Geometry check sheet. Reference: the model listing, model coordinates, mm. Give positions to 0.01 mm unless a question says otherwise; leave off trailing zeros. Loops run counter-clockwise (first coordinate to the right, second up) from the corner with the lowest first, then second, coordinate; pieces in that order, holes last.
1. Cross-section at C-C, the plane x = 16.5. Record the cut outline in (y, z), plus the area to 3 significant figures.
2. Cross-section at A-A, the plane y = 11. Record the cut outline in (x, z), plus the area to 3 significant figures.
3. Cross-section at B-B, the plane x = 28. Record the cut outline in (y, z).
4. Release check for a two-part mould opening along Y. For faces 1 (the cylindrical face through (28.378, 21.699, 4.715)), 2 (the flat face through (27.6, 13.4, 5)), 3 (the flat face through (28, 0, 2)), 4 (the cylindrical face through (39.24, 12.983, 2.535)) record: +Y half, -Y half, draft (parallel to the pull), parting line (faces both ways), or undercut.
5. Material ranges on L1, parallel to Y at x = 16.5, z = 1.45; L2, parallel to X at y = 10.5, z = 3.3; L3, parallel to Y at x = 6, z = 4.1, recorded low to high.
6. Cross-section at D-D, the plane x = 40.5. Record the cut outline in (y, z).
from build123d import *

# Parameters (mm, degrees)
SKETCH_BASE_W                                   = 56
SKETCH_BASE_H                                   = 22
BASE_EXTRUDE_DEPTH                              = 5
SKETCH2_R                                       = 2
MOUNTING_HOLES_DEPTH                            = 61.373835392
SMALL_EDGE_FILLET_R                             = 1
FILLET4_R                                       = 1
CSK_FOR_M4_FLAT_HEAD_MACHINE_SCREW4_D           = 4.3
CSK_FOR_M4_FLAT_HEAD_MACHINE_SCREW4_CSINK_D     = 9.4
CSK_FOR_M4_FLAT_HEAD_MACHINE_SCREW4_CSINK_ANGLE = 90


with BuildPart() as part:
    # Sketch-Base → Base-Extrude (new body)
    with BuildSketch(Plane.XY):
        with Locations((28, 11)):
            Rectangle(SKETCH_BASE_W, SKETCH_BASE_H)
    extrude(amount=BASE_EXTRUDE_DEPTH)

    # Sketch2 → Mounting Holes (cut, through all)
    with BuildSketch(Plane.XY.offset(5)):
        with Locations((16.5, 11)):
            Circle(SKETCH2_R)
        with Locations((39.5, 11)):
            Circle(SKETCH2_R)
    extrude(amount=-MOUNTING_HOLES_DEPTH, mode=Mode.SUBTRACT)

    # Small Edge Fillet
    small_edge_fillet_edges = [part.edges().sort_by_distance(p)[0] for p in [
        (0, 22, 2.5),
        (56, 22, 2.5),
        (56, 0, 2.5),
        (0, 0, 2.5),
    ]]
    fillet(small_edge_fillet_edges, radius=SMALL_EDGE_FILLET_R)

    # Fillet4
    fillet4_edges = [part.edges().sort_by_distance(p)[0] for p in [
        (28, 22, 0),
        (28, 22, 5),
        (0, 11, 0),
        (56, 11, 0),
        (28, 0, 0),
        (0.292893219, 21.707106781, 0),
        (0.292893219, 0.292893219, 0),
        (55.707106781, 0.292893219, 0),
        (55.707106781, 21.707106781, 0),
        (56, 11, 5),
        (0, 11, 5),
        (28, 0, 5),
        (0.292893219, 21.707106781, 5),
        (0.292893219, 0.292893219, 5),
        (55.707106781, 0.292893219, 5),
        (55.707106781, 21.707106781, 5),
    ]]
    fillet(fillet4_edges, radius=FILLET4_R)

    # CSK for M4 Flat Head Machine Screw4 (through all)
    with Locations(Plane(origin=(28, 11, 0), x_dir=(-1, 0, 0), z_dir=(0, 0, -1))):
        with Locations((0, 0)):
            CounterSinkHole(CSK_FOR_M4_FLAT_HEAD_MACHINE_SCREW4_D / 2, CSK_FOR_M4_FLAT_HEAD_MACHINE_SCREW4_CSINK_D / 2, counter_sink_angle=CSK_FOR_M4_FLAT_HEAD_MACHINE_SCREW4_CSINK_ANGLE)


solid = part.part
Result:
1. outline: (0, 1) arc R1 ccw to (1, 0) - (9, 0) - (9, 5) - (1, 5) arc R1 ccw to (0, 4) - close; (13, 0) - (21, 0) arc R1 ccw to (22, 1) - (22, 4) arc R1 ccw to (21, 5) - (13, 5) - close
1. area: 89.1 mm2
2. outline: (0, 1) arc R1 ccw to (1, 0) - (14.5, 0) - (14.5, 5) - (1, 5) arc R1 ccw to (0, 4) - close; (18.5, 0) - (23.3, 0) - (25.85, 2.55) - (25.85, 5) - (18.5, 5) - close; (30.15, 2.55) - (32.7, 0) - (37.5, 0) - (37.5, 5) - (30.15, 5) - close; (41.5, 0) - (55, 0) arc R1 ccw to (56, 1) - (56, 4) arc R1 ccw to (55, 5) - (41.5, 5) - close
2. area: 211 mm2
3. outline: (0, 1) arc R1 ccw to (1, 0) - (6.3, 0) - (8.85, 2.55) - (8.85, 5) - (1, 5) arc R1 ccw to (0, 4) - close; (13.15, 2.55) - (15.7, 0) - (21, 0) arc R1 ccw to (22, 1) - (22, 4) arc R1 ccw to (21, 5) - (13.15, 5) - close
4. face 1: +Y half
4. face 2: draft
4. face 3: -Y half
4. face 4: undercut
5. L1: y = 0 to 9, 13 to 22
5. L2: x = 0 to 14.56, 18.44 to 25.91, 30.09 to 37.56, 41.44 to 56
5. L3: y = 0.01 to 21.99
6. outline: (0, 1) arc R1 ccw to (1, 0) - (9.27, 0) - (9.27, 5) - (1, 5) arc R1 ccw to (0, 4) - close; (12.73, 0) - (21, 0) arc R1 ccw to (22, 1) - (22, 4) arc R1 ccw to (21, 5) - (12.73, 5) - close
